```python
from build123d import *

# Parameters (mm, degrees)
F0_W     = 500
F0_H     = 500
F0_R     = 25
F1_DEPTH = 19
F2_W     = 500
F2_H     = 500
F2_W_2   = 462
F2_H_2   = 462
F2_W_3   = 120
F2_H_3   = 120
F2_R     = 25
F3_DEPTH = 50
F4_SIZE  = 10


with BuildPart() as f1:
    # F0 (on Top) → F1 (new body)
    with BuildSketch(Plane.XY):
        Rectangle(F0_W, F0_H)
        Circle(F0_R, mode=Mode.SUBTRACT)
    extrude(amount=F1_DEPTH)

    # F2 (on face) → F3 (join)
    with BuildSketch(Plane(origin=(0, 0, 0), x_dir=(1, 0, 0), z_dir=(0, 0, -1))):
        Rectangle(F2_W, F2_H)
        Rectangle(F2_W_2, F2_H_2, mode=Mode.SUBTRACT)
        Rectangle(F2_W_3, F2_H_3)
        Circle(F2_R, mode=Mode.SUBTRACT)
    extrude(amount=F3_DEPTH)

    # F4
    f4_edges = [f1.edges().sort_by_distance(p)[0] for p in [
        (0, 250, 19),
        (250, 0, 19),
        (0, -250, 19),
        (-250, 0, 19),
        (-250, 250, -15.5),
        (-250, -250, -15.5),
        (250, 250, -15.5),
        (250, -250, -15.5),
    ]]
    chamfer(f4_edges, length=F4_SIZE)


solid = f1.part
```
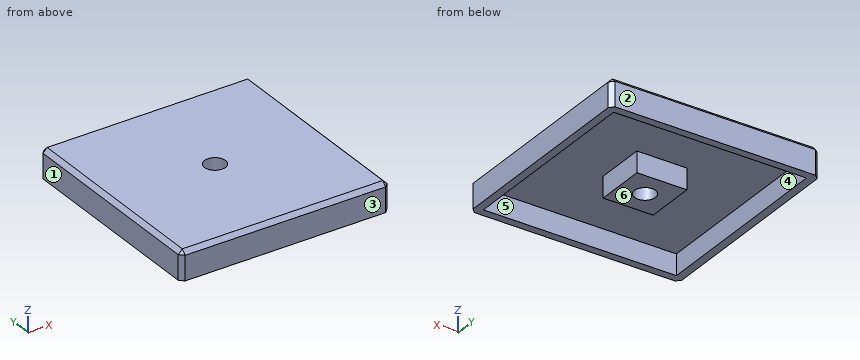
Check sheet for the modelled part. Datum: model origin and axes. Units: mm. Face numbers are marked on the shaded views. A direction names the side the tool comes from. Round coordinates to 2 decimals unless told otherwise and drop trailing zeros. Write each loop counter-clockwise with the first axis right and the second up, starting at its lowest first coordinate (ties: lowest second). Pieces come first, ordered by that corner, then holes. Notation, with made-up numbers: (-31, -9) -> (4, -9) arc R20 ccw to (4, 14) -> close; hole circle Ø2 at (-36.75, 71). An arc over 180 degrees is marked (long way). One line per question, with ' | ' between items. Start each with the question number.
1. Release check for a two-part mould opening along Y. For the marked faces 1, 2, 3 and 4 record: +Y half, -Y half, draft (parallel to the pull), parting line (faces both ways), or undercut.
2. Sectioned sample at A-A, the plane z = -27. Record the cut outline in (x, y), then the cut area to 3 significant figures.
3. Set-up check for the marked faces 5 and 6: record each of +Z, -Z, +X, -X, +Y, -Y from which the full face is reachable in a straight line by a thin tool's end or side.
4. Sectioned sample at D-D, the plane y = -116. Record the cut outline in (x, z).
5. Sectioned sample at B-B, the plane x = 0. Record the cut outline in (y, z), then the cut area to 4 significant figures.
6. Scan lines: line 1 along Y through (x, z) = (0, -12.5); line 2 along Y through (x, z) = (-31.5, -39). Record each from-to range of solid material in increasing order. Write a range as from..to.
Taken from the geometry:
1) face 1: draft | face 2: +Y half | face 3: -Y half | face 4: undercut
2) outline: (-250, -240) -> (-240, -250) -> (240, -250) -> (250, -240) -> (250, 240) -> (240, 250) -> (-240, 250) -> (-250, 240) -> close; (-60, -60) -> (60, -60) -> (60, 60) -> (-60, 60) -> close; hole (-231, -231) -> (231, -231) -> (231, 231) -> (-231, 231) -> close; hole circle Ø50 at (0, 0) | area: 48,800 mm^2
3) face 5: -Z | face 6: -Z, +X, -X, +Y, -Y
4) outline: (-250, -50) -> (-231, -50) -> (-231, 0) -> (231, 0) -> (231, -50) -> (250, -50) -> (250, 9) -> (240, 19) -> (-240, 19) -> (-250, 9) -> close
5) outline: (-250, -50) -> (-231, -50) -> (-231, 0) -> (-60, 0) -> (-60, -50) -> (-25, -50) -> (-25, 19) -> (-240, 19) -> (-250, 9) -> close; (25, -50) -> (60, -50) -> (60, 0) -> (231, 0) -> (231, -50) -> (250, -50) -> (250, 9) -> (240, 19) -> (25, 19) -> close | area: 13,850 mm^2
6) line 1: y = -250..-231, -60..-25, 25..60, 231..250 | line 2: y = -250..-231, -60..60, 231..250
